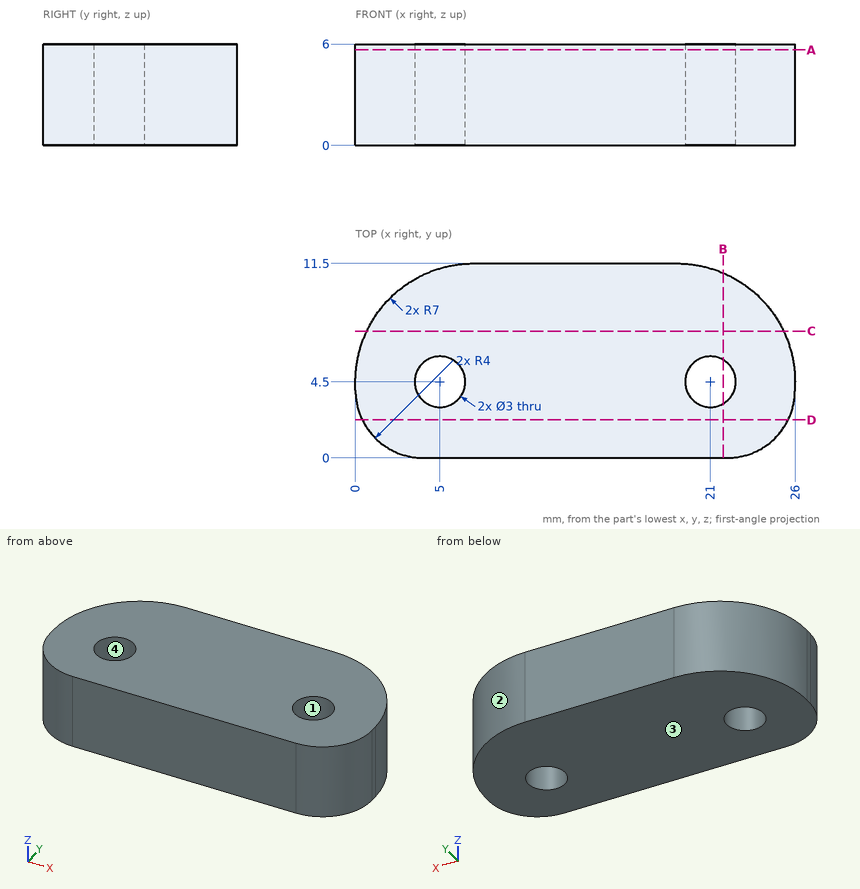
The drawing under review shows one solid part. Ordinate dimensions are in mm from its lowest x, y, z. Coordinates: 2 decimals unless noted, no trailing zeros. Write each loop counter-clockwise with the first axis right and the second up, starting at its lowest first coordinate (ties: lowest second). Pieces come first, ordered by that corner, then holes.
1) Add section A-A (z = 5.65). Write out the cut boundary in (x, y).
2) Add section B-B (x = 21.75). Write out the cut boundary in (y, z), plus the area to 3 significant figures.
3) To check wall thickness, follow L1, parallel to X at y = 4.25, z = 5.2; L2, parallel to X at y = 5, z = 1.4; L3, parallel to X at y = 9, z = 1. State the ranges of each line that lie inside material, in increasing order.
4) Add section D-D (y = 2.25). Write out the cut boundary in (x, z).
5) Mouldability with a two-part tool opening along Y and no side actions: class the marked faces 1, 2, 3 and 4 as +Y half, -Y half, draft (parallel to the pull), parting line (faces both ways), or undercut.
6) Add section C-C (y = 7.5). Write out the cut boundary in (x, z), plus the area to 3 significant figures.
7) Insertion check: pin 1 (1.5 mm diameter, centred on y = 2, z = 2, fed in from -X); pin 2 (2.5 mm diameter, centred on x = 21, y = 4.5, fed in from -Z); pin 3 (4 mm diameter, centred on x = 5, y = 4.5, fed in from -Z); pin 4 (2 mm diameter, centred on y = 7.5, z = 3, fed in from +X). Each pin has a flat end and moves straight along its axis. Give the tip position at first contact, or say it passes through.
Check result:
1. outline: (0, 4) arc R4 ccw to (4, 0) - (22, 0) arc R4 ccw to (26, 4) - (26, 4.5) arc R7 ccw to (19, 11.5) - (7, 11.5) arc R7 ccw to (0, 4.5) - close; hole circle Ø3 at (5, 4.5); hole circle Ø3 at (21, 4.5)
2. outline: (0, 0) - (3.2, 0) - (3.2, 6) - (0, 6) - close; (5.8, 0) - (10.94, 0) - (10.94, 6) - (5.8, 6) - close
2. area: 50.0 mm2
3. L1: x = 0 to 3.52, 6.48 to 19.52, 22.48 to 26
3. L2: x = 0.02 to 3.59, 6.41 to 19.59, 22.41 to 25.98
3. L3: x = 1.64 to 24.36
4. outline: (0.4, 0) - (25.6, 0) - (25.6, 6) - (0.4, 6) - close
5. face 1: undercut
5. face 2: +Y half
5. face 3: draft
5. face 4: undercut
6. outline: (0.68, 0) - (25.32, 0) - (25.32, 6) - (0.68, 6) - close
6. area: 148 mm2
7. pin 1: stops at x = 0.2
7. pin 2: passes through
7. pin 3: stops at z = 0
7. pin 4: stops at x = 25.71
